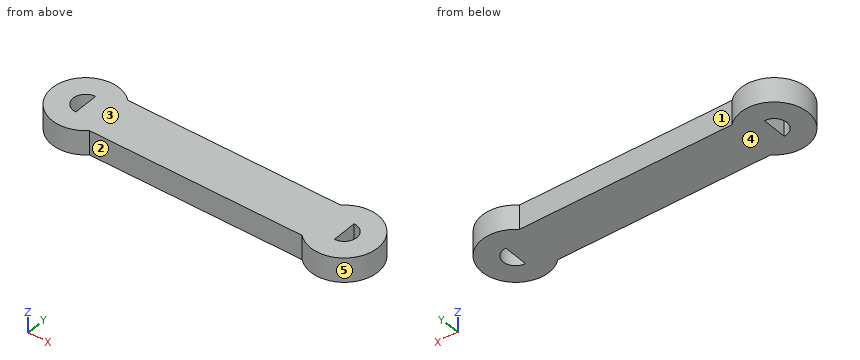
```python
from build123d import *

# Parameters (mm, degrees)
SKETCH_1_W      = 85
SKETCH_1_H      = 16
EXTRUDE_1_DEPTH = 8
SKETCH_2_R      = 11
SKETCH_2_R_2    = 4.1
EXTRUDE_2_DEPTH = 8
SKETCH_3_R      = 11
SKETCH_3_R_2    = 4.1
EXTRUDE_3_DEPTH = 8


with BuildPart() as part:
    # 草图1 → 凸台-拉伸1 (new body)
    with BuildSketch(Plane.XY):
        with Locations((42.5, 0)):
            Rectangle(SKETCH_1_W, SKETCH_1_H)
    extrude(amount=EXTRUDE_1_DEPTH)

    # 草图2 → 凸台-拉伸2 (add)
    with BuildSketch(Plane.XY):
        Circle(SKETCH_2_R)
        Circle(SKETCH_2_R_2, mode=Mode.SUBTRACT)
    extrude(amount=EXTRUDE_2_DEPTH)

    # 草图3 → 凸台-拉伸3 (add)
    with BuildSketch(Plane.XY):
        with Locations((85, 0)):
            Circle(SKETCH_3_R)
        with Locations((85, 0)):
            Circle(SKETCH_3_R_2, mode=Mode.SUBTRACT)
    extrude(amount=EXTRUDE_3_DEPTH)


solid = part.part
```
Design review of the part built by this model. Coordinates are the model's own, in mm. Face numbers are marked on the shaded views. A direction names the side the tool comes from. Round coordinates to 2 decimals unless told otherwise and drop trailing zeros. Order: outer loops, then holes, each group sorted by start corner. A loop starts at its lowest first (then second) coordinate and runs counter-clockwise, first axis right, second up. Notation, with made-up numbers: (43.25, 53) - (49.25, 53) arc R10 cw to (49.25, 68) - close; hole circle Ø9 at (-26.5, 67). An arc over 180 degrees is marked (long way). Return JSON: item names as keys, results as strings.
Q1. For pin 1 Ø1.5 at (y, z) = (-5, 3.5) entering from +X; pin 2 Ø2.5 at (x, z) = (26, 4) entering from +Y; pin 3 Ø2.5 at (x, z) = (28, 4.5) entering from -Y, all flat-tipped, find the tip position at first contact; note any pin that passes through.
Computed values:
{"pin 1": "stops at x = 95.15", "pin 2": "stops at y = 8", "pin 3": "stops at y = -8"}
Q2. The part is to be moulded in two halves that separate along X. For the marked faces 4 and 5, say which applies: pulls with the +X half, pulls with the -X half, needs draft (parallel to the pull), parting line crosses it, or undercut.
Computed values:
{"face 4": "needs draft", "face 5": "undercut"}
Q3. Consider section B-B on z = 2.5. Write out the cut boundary in (x, y), plus the area to 3 significant figures.
Computed values:
{"outline": "(7.55, -8) - (77.45, -8) arc R11 ccw (long way) to (77.45, 8) - (7.55, 8) arc R11 ccw (long way) to start; hole (0, -4.1) - (0, 4.1) arc R4.1 ccw to start; hole (85, -4.1) arc R4.1 ccw to (85, 4.1) - close", "area": "1,750 mm2"}
Q4. Consider section A-A on y = 0. Write out the cut boundary in (x, z), plus the area to 3 significant figures.
Computed values:
{"outline": "(-11, 0) - (-4.1, 0) - (-4.1, 8) - (-11, 8) - close; (0, 0) - (85, 0) - (85, 8) - (0, 8) - close; (89.1, 0) - (96, 0) - (96, 8) - (89.1, 8) - close", "area": "790 mm2"}
Q5. Wall thickness on L1, parallel to X at y = 3.25, z = 5; L2, parallel to X at y = -0.75, z = 0.5; L3, parallel to Y at x = 43, z = 3: over which ranges is each line inside the solid? List them lowest first. Write a range as [from, to].
Computed values:
{"L1": "x = [-10.51, -2.5], [0, 85], [87.5, 95.51]", "L2": "x = [-10.97, -4.03], [0, 85], [89.03, 95.97]", "L3": "y = [-8, 8]"}
Q6. Machinability: for the marked faces 1, 2 and 3, which of the approach directions +Z, -Z, +X, -X, +Y, -Y give a long, thin tool a straight path to every point of the face, cutting with its end or side? Answer none if there is none.
Computed values:
{"face 1": "+Z, -Z, +Y", "face 2": "+Z, -Z, -Y", "face 3": "+Z, +X, -X, +Y, -Y"}
